Verification items for the finished model (mm, model axes). Face numbers are marked on the shaded views. A direction names the side the tool comes from. Coordinates: 2 decimals unless noted, no trailing zeros. Loops run counter-clockwise (first coordinate to the right, second up) from the corner with the lowest first, then second, coordinate; pieces in that order, holes last.
Q1. Sectioned sample at A-A (y = 14.25). Enter the section's corners in (x, z), then the cut area to 3 significant figures.
Q2. Go/stop test with flat-tipped pins: P1, Ø1.2, axis at x = 10.5, z = 1, coming from the +Y side; P2, Ø1.2, axis at x = -11.5, y = 20.5, coming from the -Z side; P3, Ø1.5, axis at x = -28, z = 1.5, coming from the -Y side; P4, Ø1.5, axis at x = -31, z = 8.5, coming from the +Y side. Record where each tip stops, or that it passes through.
Q3. Sectioned sample at D-D (y = 18.75). Count the separate pieces of the cut face and the enclosed holes in it, then the cut area to 3 significant figures.
Q4. Sectioned sample at B-B (x = 7.5). Enter the section's corners in (y, z), then the cut area to 3 significant figures.
Q5. Access from +Z, -Z, +X, -X, +Y, -Y to the whole of each face (thin tool, end or side, straight path). Record for the marked faces 4 and 5.
Q6. Sectioned sample at C-C (z = 6). Enter the section's corners in (x, y), then the cut area to 3 significant figures.
Q7. Mould release check, pull along X, two halves, no side actions. Record for the marked faces 1, 2 and 3: +X half, -X half, draft (parallel to the pull), parting line (faces both ways), or undercut.
Q8. Material ranges on probe 1 along X at (y, z) = (20.75, 5.5); probe 2 along Y at (x, z) = (-0.5, 1.25); probe 3 along Y at (x, z) = (-29.5, 5.5), recorded low to high.
```python
from build123d import *

# Parameters (mm, degrees)
SALIENTE_EXTRUIR1_DEPTH = 14
CROQUIS2_W              = 8.5
CROQUIS2_H              = 3
SALIENTE_EXTRUIR2_DEPTH = 4
SALIENTE_EXTRUIR3_DEPTH = 4
REDONDEO1_R             = 3


with BuildPart() as part:
    # Croquis1 → Saliente-Extruir1 (new body)
    with BuildSketch(Plane.XY):
        with BuildLine():
            Line((-38.5, 7.5), (-41, 7.5))
            Line((-41, 7.5), (-41, 17.5))
            Line((-41, 17.5), (41, 17.5))
            Line((41, 17.5), (41, 7.5))
            Line((41, 7.5), (38.5, 7.5))
            Line((38.5, 7.5), (38.5, 12))
            Line((38.5, 12), (35, 12))
            ThreePointArc((35, 12), (32.354101966, 14.208203932), (29, 15))
            Line((29, 15), (-31, 15))
            ThreePointArc((-31, 15), (-36.303300859, 12.803300859), (-38.5, 7.5))
        make_face()
    extrude(amount=SALIENTE_EXTRUIR1_DEPTH)

    # Croquis2 → Saliente-Extruir2 (add)
    with BuildSketch(Plane.XY):
        with Locations((29, 19)):
            Rectangle(CROQUIS2_W, CROQUIS2_H)
        with Locations((-31, 19)):
            Rectangle(CROQUIS2_W, CROQUIS2_H)
        with Locations((-11, 19)):
            Rectangle(CROQUIS2_W, CROQUIS2_H)
        with Locations((9, 19)):
            Rectangle(CROQUIS2_W, CROQUIS2_H)
    extrude(amount=SALIENTE_EXTRUIR2_DEPTH)

    # Croquis3 → Saliente-Extruir3 (add)
    with BuildSketch(Plane(origin=(0, 17.5, 0), x_dir=(1, 0, 0), z_dir=(0, 1, 0))):
        Polygon((-41, -14), (41, -14), (41, 0), (36.75, 0), (36.75, -11), (21.25, -11), (21.25, 0), (16.75, 0), (16.75, -11), (1.25, -11), (1.25, 0), (-3.25, 0), (-3.25, -11), (-18.75, -11), (-18.75, 0), (-23.25, 0), (-23.25, -11), (-38.75, -11), (-38.75, 0), (-41, 0), align=None)
    extrude(amount=SALIENTE_EXTRUIR3_DEPTH)

    # Redondeo1
    redondeo1_edges = [part.edges().sort_by_distance(p)[0] for p in [
        (-41, 14.5, 14),
        (41, 14.5, 14),
    ]]
    fillet(redondeo1_edges, radius=REDONDEO1_R)


solid = part.part
```
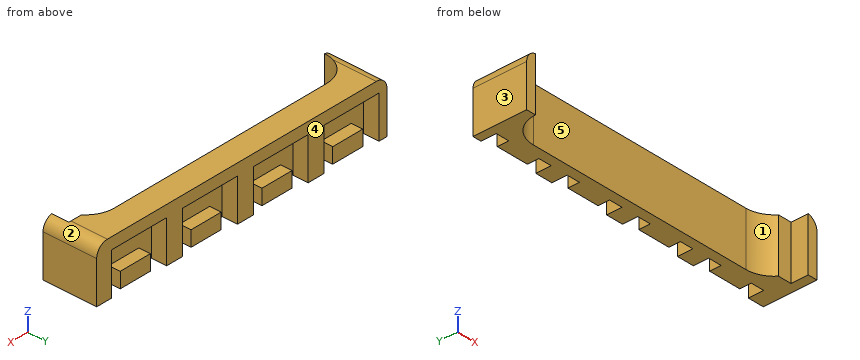
Geometry check:
1. outline: (-41, 0) - (-34.27, 0) - (-34.27, 14) - (-38, 14) arc R3 ccw to (-41, 11) - close; (32.27, 0) - (41, 0) - (41, 11) arc R3 ccw to (38, 14) - (32.27, 14) - close
1. area: 213 mm2
2. P1: stops at y = 20.5
2. P2: stops at z = 0
2. P3: stops at y = 15
2. P4: stops at y = 17.5
3. separate pieces: 5
3. enclosed holes: 0
3. area: 598 mm2
4. outline: (15, 0) - (20.5, 0) - (20.5, 4) - (17.5, 4) - (17.5, 11) - (21.5, 11) - (21.5, 14) - (15, 14) - close
4. area: 59.0 mm2
5. face 4: +Z, -Z, +X, -X, +Y
5. face 5: +Z, -Z, -Y
6. outline: (-41, 7.5) - (-38.5, 7.5) arc R7.5 cw to (-31, 15) - (29, 15) arc R7.5 cw to (35, 12) - (38.5, 12) - (38.5, 7.5) - (41, 7.5) - (41, 21.5) - (36.75, 21.5) - (36.75, 17.5) - (21.25, 17.5) - (21.25, 21.5) - (16.75, 21.5) - (16.75, 17.5) - (1.25, 17.5) - (1.25, 21.5) - (-3.25, 21.5) - (-3.25, 17.5) - (-18.75, 17.5) - (-18.75, 21.5) - (-23.25, 21.5) - (-23.25, 17.5) - (-38.75, 17.5) - (-38.75, 21.5) - (-41, 21.5) - close
6. area: 350 mm2
7. face 1: undercut
7. face 2: +X half
7. face 3: -X half
8. probe 1: x = -41 to -38.75, -23.25 to -18.75, -3.25 to 1.25, 16.75 to 21.25, 36.75 to 41
8. probe 2: y = 15 to 21.5
8. probe 3: y = 15 to 17.5
